Autodesk Fusion 360 part; units mm, degrees
sketch "Sketch1" plane through (0, 0, 0) normal (0, 1, 0) x (1, 0, 0)
  circle A0 centre (0, 0) radius 5
  dimension "d1" = 10
extrude "Extrude1" add sketch "Sketch1" along normal blind 33
chamfer "Chamfer1" distance 5 angle 45 1 edges at (-4.6616, 0, 1.8081)
ref_plane "WorkPlane1" through (0, 0, -5) normal (0, 0, 1) x (1, 0, 0)
sketch "Sketch2" plane through (0, 0, -5) normal (0, 0, 1) x (1, 0, 0)
sketch "Sketch3" plane through (0, 33, 0) normal (0, 1, 0) x (-1, 0, 0)
  circle A0 centre (0, 0) radius 5
  line L0 (0, 0) -> (0.8, 0)
  line L1 (0, 0) -> (-0.8, 0)
  line L2 (-0.8, 0) -> (-0.8, 5.3819)
  line L3 (0.8, 0) -> (0.8, 5.3174)
  line L4 (0.8, 5.3174) -> (-0.8, 5.3819)
  line L5 (0.8, 0) -> (0.8, -5.6853)
  line L6 (-0.8, 0) -> (-0.8, -5.7176)
  line L7 (-0.8, -5.7176) -> (0.8, -5.6853)
  dimension "d6" = 0.8
  dimension "d7" = 0.8
extrude "Extrude2" cut sketch "Sketch3" against normal blind 3 contours A0 L0 L1 L2 L3 | A0 L0 L1 L5 L6
Can you work these out from the model? Positions are in its coordinate system, mm. A direction names the side the tool comes from. Give positions to 0.01 mm unless a question says otherwise; leave off trailing zeros. Order: outer loops, then holes, each group sorted by start corner. A loop starts at its lowest first (then second) coordinate and runs counter-clockwise, first axis right, second up. Notation, with made-up numbers: (14.5, -22.75) - (25.5, -22.75) arc R15 cw to (25.5, 6.25) - close; hole circle Ø11 at (39.25, 87). An arc over 180 degrees is marked (long way). Write each question's results on one line, items separated by ' | '.
1) If we mould it in two halves opening along X, with no side actions, what happens to faces 1 (the face through (2, 33, 0)), 2 (the face through (-1.08, 18.8, -4.88)), 3 (the face through (-0.8, 32, 0))? For each: pulls with the +X half, pulls with the -X half, needs draft (parallel to the pull), parting line crosses it, or undercut.
Final values:
face 1: needs draft | face 2: parting line crosses it | face 3: undercut
2) Please list where these lines run through material, in increasing order: line 1 along X through (y, z) = (29, -0.75); line 2 along Y through (x, z) = (2.5, -4.25); line 3 along Z through (x, y) = (0.25, 13.5). Write a range as [from, to].
Final values:
line 1: x = [-4.94, 4.94] | line 2: y = [4.93, 33] | line 3: z = [-4.99, 4.99]
3) Suppose I cut it at A-A, the plane y = 12. Write out the boundary of the cut face in (x, z), then the cut area to 3 significant figures.
Final values:
outline: circle Ø10 at (0, 0) | area: 78.5 mm^2
4) I'm going to push flat-ended pins straight in: pin 1 Ø1 at (x, y) = (3.5, 23.5) entering from +Z; pin 2 Ø5 at (x, z) = (-2.5, -2) entering from -Y; pin 3 Ø4 at (y, z) = (25, -2.5) entering from -X. Where does each tip first touch, or does it pass through?
Final values:
pin 1: stops at z = 4 | pin 2: stops at y = 0.7 | pin 3: stops at x = -4.97
5) On a 3-axis mill with a long thin cutter (end or side, diameter ignored), from which of +Z, -Z, +X, -X, +Y, -Y can I reach the whole of each face in a straight line? I mean faces 4 (the face through (-2, 33, 0)), 5 (the face through (0, 30, 0)). Say none if no direction works.
Final values:
face 4: +Z, -Z, +X, -X, +Y | face 5: +Z, -Z, +Y
